Design review of the part built by this model. Coordinates are the model's own, in mm. A direction names the side the tool comes from. Round coordinates to 2 decimals unless told otherwise and drop trailing zeros. Write each loop counter-clockwise with the first axis right and the second up, starting at its lowest first coordinate (ties: lowest second). Pieces come first, ordered by that corner, then holes.
from build123d import *

# Parameters (mm, degrees)
BOSS_EXTRUDE1_DEPTH      = 18.7
FILLET1_R                = 5
FILLET2_R                = 2
CHAMFER1_SIZE            = 3
SKETCH2_R                = 3
SKETCH2_R_2              = 0.9
CUT_EXTRUDE1_DEPTH       = 18.7
SKETCH3_R                = 0.414419125
CUT_EXTRUDE2_DEPTH       = 118.7
BOSS_EXTRUDE2_DEPTH      = 25
BOSS_EXTRUDE2_DEPTH_BACK = 5
SKETCH4_R                = 2.75
CHAMFER2_SIZE            = 5
FILLET3_R                = 1


with BuildPart() as part:
    # Sketch1 → Boss-Extrude1 (new body)
    with BuildSketch(Plane.XY):
        Polygon((-45, -16.035242291), (45, -16.035242291), (45, 23.964757709), (50, 23.964757709), (50, -16.035242291), (50, -21.035242291), (-50, -21.035242291), (-50, -16.035242291), (-50, 23.964757709), (-45, 23.964757709), align=None)
    extrude(amount=BOSS_EXTRUDE1_DEPTH)

    # Fillet1
    fillet1_edges = [part.edges().sort_by_distance(p)[0] for p in [
        (47.5, 23.964757709, 18.7),
        (-47.5, 23.964757709, 0),
        (47.5, 23.964757709, 0),
        (-47.5, 23.964757709, 18.7),
    ]]
    fillet(fillet1_edges, radius=FILLET1_R)

    # Fillet2
    fillet2_edges = [part.edges().sort_by_distance(p)[0] for p in [
        (-45, -16.035242291, 9.35),
        (45, -16.035242291, 9.35),
    ]]
    fillet(fillet2_edges, radius=FILLET2_R)

    # Chamfer1
    chamfer1_edges = [part.edges().sort_by_distance(p)[0] for p in [
        (50, -21.035242291, 9.35),
        (-50, -21.035242291, 9.35),
    ]]
    chamfer(chamfer1_edges, length=CHAMFER1_SIZE)

    # Sketch2 → Cut-Extrude1 (cut)
    with BuildSketch(Plane.ZY.offset(50)):
        with Locations((9.35, 13.964757709)):
            Circle(SKETCH2_R)
        with Locations((9.35, 20.964757709)):
            Circle(SKETCH2_R_2)
        with Locations((9.35, 6.964757709)):
            Circle(SKETCH2_R_2)
    extrude(amount=-CUT_EXTRUDE1_DEPTH, mode=Mode.SUBTRACT)

    # Sketch3 → Cut-Extrude2 (cut)
    with BuildSketch(Plane.ZY.offset(50)):
        with Locations((9.35, 13.964757709)):
            Circle(SKETCH3_R)
    extrude(amount=-CUT_EXTRUDE2_DEPTH, mode=Mode.SUBTRACT)

    # Sketch4 → Boss-Extrude2 (add, two sides: drawn at the far end of the back side and taken through both)
    with BuildSketch(Plane(origin=(50, 0, 0), x_dir=(0, 0, -1), z_dir=(1, 0, 0)).offset(-BOSS_EXTRUDE2_DEPTH_BACK)):
        with Locations((-9.35, 13.964757709)):
            Circle(SKETCH4_R)
    extrude(amount=BOSS_EXTRUDE2_DEPTH + BOSS_EXTRUDE2_DEPTH_BACK)

    # Chamfer2
    chamfer2_edges = [part.edges().sort_by_distance(p)[0] for p in [
        (50, 13.964757709, 12.1),
    ]]
    chamfer(chamfer2_edges, length=CHAMFER2_SIZE)

    # Fillet3
    fillet3_edges = [part.edges().sort_by_distance(p)[0] for p in [
        (75, 13.964757709, 12.1),
    ]]
    fillet(fillet3_edges, radius=FILLET3_R)


solid = part.part
1) The part is to be moulded in two halves that separate along Z. For faces 1 (the face through (0, -19, 18.7)), 2 (the face through (-47.535, 15.992, 7.139)), 3 (the face through (50, -2, 9)), 4 (the face through (64.37, 12.91, 6.81)), say which applies: pulls with the +Z half, pulls with the -Z half, needs draft (parallel to the pull), parting line crosses it, or undercut.
2) Add section A-A on y = -11. State the section outline as (x, z) points, and give its area (3 significant figures).
3) For faces 5 (the face through (0, -19, 0)), 6 (the face through (-45, 5, 9)), list the 3-axis set-ups (+Z, -Z, +X, -X, +Y, -Y) from which the entire face can be reached by the end or side of a thin tool; tool diameter is ignored.
4) For P1, Ø1, axis at x = 6.5, z = 7, coming from the +Y side; P2, Ø1.4, axis at y = 20.96, z = 9.35, coming from the +X side; P3, Ø6, axis at x = 61, z = 5.5, coming from the +Y side, all flat-tipped, find the tip position at first contact; note any pin that passes through.
5) Add section B-B on x = -7. State the section outline as (y, z) points.
6) For line 1 along Y through (x, z) = (-46.65, 9.35); line 2 along X through (y, z) = (5, 13.5); line 3 along Y through (x, z) = (-48.5, 9.35), list the stretches that pass through material, from the lowest coordinate up.
Computed:
1. face 1: pulls with the +Z half
1. face 2: undercut
1. face 3: needs draft
1. face 4: parting line crosses it
2. outline: (-50, 0) - (-45, 0) - (-45, 18.7) - (-50, 18.7) - close; (45, 0) - (50, 0) - (50, 18.7) - (45, 18.7) - close
2. area: 187 mm2
3. face 5: -Z, +X, -X, +Y, -Y
3. face 6: +Z, -Z, +Y
4. P1: stops at y = -16.04
4. P2: stops at x = 51.45
4. P3: stops at y = 16.58
5. outline: (-21.04, 0) - (-16.04, 0) - (-16.04, 18.7) - (-21.04, 18.7) - close
6. line 1: y = -21.04 to 6.06, 7.86 to 10.96, 16.96 to 20.06, 21.86 to 23.96
6. line 2: x = -50 to -45, 45 to 50
6. line 3: y = -19.54 to 6.06, 7.86 to 10.96, 16.96 to 20.06, 21.86 to 23.96
